Geometry check sheet. Reference: the model listing, model coordinates, mm. Face numbers are marked on the shaded views. A direction names the side the tool comes from. Coordinates: 2 decimals unless noted, no trailing zeros. Write each loop counter-clockwise with the first axis right and the second up, starting at its lowest first coordinate (ties: lowest second). Pieces come first, ordered by that corner, then holes. Notation, with made-up numbers: M 65,-8.5 L 102,-8.5 A15 cw 102,5.5 Z; hole C 19.5,-7.75 d3. An arc over 180 degrees is marked long. Put each result on its own line as item: value. Start each with the question number.
1) Gauge pin test, flat ends, axial feed: pin 1 (1 mm diameter, centred on x = 0.5, z = 16.5, fed in from +Y); pin 2 (1 mm diameter, centred on x = 1.5, z = -15.5, fed in from +Y); pin 3 (1.4 mm diameter, centred on x = 1, z = -21.5, fed in from +Y). Record the tip position at first contact, or that the pin passes through.
2) Cross-section at A-A on z = -19.5. Record the cut outline in (x, y).
3) Set-up check for the marked faces 1, 2 and 3: record each of +Z, -Z, +X, -X, +Y, -Y from which the full face is reachable in a straight line by a thin tool's end or side.
4) Cross-section at B-B on z = -3.5. Record the cut outline in (x, y), plus the area to 3 significant figures.
5) Scan lines: line 1 along Y through (x, z) = (-1.25, -20); line 2 along X through (y, z) = (1, 3); line 3 along Z through (x, y) = (1.8, 1.45). Record each from-to range of solid material in increasing order.
6) Cross-section at C-C on z = 11.5. Record the cut outline in (x, y), plus the area to 3 significant figures.
from build123d import *

# Parameters (mm, degrees)
SKETCH1_R           = 2.5
BOSS_EXTRUDE1_DEPTH = 25
SKETCH2_R           = 3
BOSS_EXTRUDE2_DEPTH = 11
CHAMFER1_SIZE2      = 0.5
CHAMFER1_SIZE       = 0.866025404
BOSS_EXTRUDE3_START = 5
SKETCH3_R           = 2.5
BOSS_EXTRUDE3_DEPTH = 5
CHAMFER3_SIZE2      = 0.866025404
CHAMFER3_SIZE       = 0.5
BOSS_EXTRUDE4_START = 7.85
BOSS_EXTRUDE4_DEPTH = 7.85


with BuildPart() as part:
    # Sketch1 → Boss-Extrude1 (new body)
    with BuildSketch(Plane.XY):
        Circle(SKETCH1_R)
    extrude(amount=BOSS_EXTRUDE1_DEPTH)

    # Sketch2 → Boss-Extrude2 (add)
    with BuildSketch(Plane(origin=(0, 0, 0), x_dir=(-1, 0, 0), z_dir=(0, 0, -1))):
        Circle(SKETCH2_R)
    extrude(amount=BOSS_EXTRUDE2_DEPTH)

    # Chamfer1
    chamfer1_edges = [part.edges().sort_by_distance(p)[0] for p in [
        (3, 0, 0),
    ]]
    chamfer1_side = [part.faces().sort_by_distance(p)[0] for p in [
        (3, 0, -0.01),
    ]]
    chamfer(chamfer1_edges, length=CHAMFER1_SIZE - 0.0001, length2=CHAMFER1_SIZE2 - 0.0001, reference=chamfer1_side[0])  # a hair under: the kernel refuses the full size

    # Sketch3 → Boss-Extrude3 (add)
    with BuildSketch(Plane(origin=(0, 0, -11), x_dir=(-1, 0, 0), z_dir=(0, 0, -1)).offset(BOSS_EXTRUDE3_START)):
        with Locations(Location((0, 0, 0), (0, 0, 180))):
            Circle(SKETCH3_R)
    extrude(amount=-BOSS_EXTRUDE3_DEPTH)

    # Chamfer3
    chamfer3_edges = [part.edges().sort_by_distance(p)[0] for p in [
        (-2.5, 0, -11),
    ]]
    chamfer3_side = [part.faces().sort_by_distance(p)[0] for p in [
        (-2.51, 0, -11),
    ]]
    chamfer(chamfer3_edges, length=CHAMFER3_SIZE - 0.0001, length2=CHAMFER3_SIZE2 - 0.0001, reference=chamfer3_side[0])  # a hair under: the kernel refuses the full size

    # Sketch4 → Boss-Extrude4 (add)
    with BuildSketch(Plane(origin=(0, 0, -16), x_dir=(-1, 0, 0), z_dir=(0, 0, -1)).offset(BOSS_EXTRUDE4_START)):
        with BuildLine():
            Line((-2.291287847, 1), (2.291287847, 1))
            ThreePointArc((2.291287847, 1), (0, -2.5), (-2.291287847, 1))
        make_face()
    extrude(amount=-BOSS_EXTRUDE4_DEPTH)

    # SurfaceCut1
    split(bisect_by=Plane(origin=(0, -2, 0), x_dir=(1, 0, 0), z_dir=(0, 1, 0)), keep=Keep.TOP)


solid = part.part
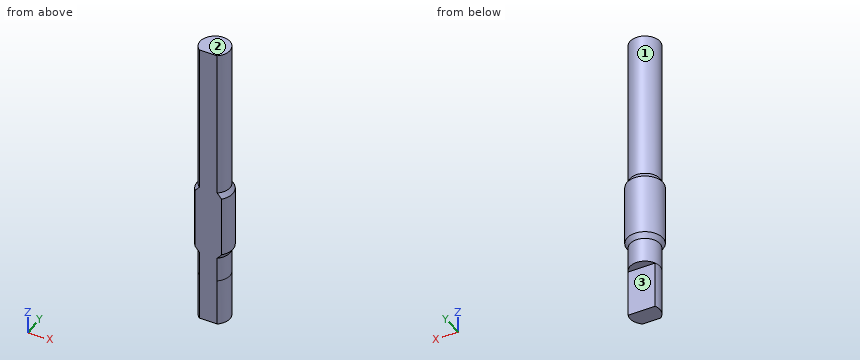
Answer key:
1. pin 1: stops at y = 2.5
1. pin 2: stops at y = 2.29
1. pin 3: stops at y = 1
2. outline: M -2.29,1 A2.5 ccw -1.5,-2 L 1.5,-2 A2.5 ccw 2.29,1 Z
3. face 1: +Z
3. face 2: +Z, +X, -X, +Y, -Y
3. face 3: -Z, +X, -X, +Y
4. outline: M -2.24,-2 L 2.24,-2 A3 ccw long Z
4. area: 25.2 mm²
5. line 1: y = -2 to 1
5. line 2: x = -2.29 to 2.29
5. line 3: z = -16 to 25
6. outline: M -1.5,-2 L 1.5,-2 A2.5 ccw long Z
6. area: 18.6 mm²
